```python
from build123d import *

# Parameters (mm, degrees)
F1_DEPTH = 20
F2_SIZE  = 5
F4_DEPTH = 25


with BuildPart() as f1:
    # F0 (on Top) → F1 (new body)
    with BuildSketch(Plane.XY):
        with BuildLine():
            Line((-45, 0), (0, 0))
            Line((0, 0), (0, 115))
            Line((0, 115), (-22, 115))
            ThreePointArc((-22, 115), (-24.12132, 115.87868), (-25, 118))
            Line((-25, 118), (-25, 120.717968))
            ThreePointArc((-25, 120.717968), (-38.514543, 135.644234), (-54.705789, 123.674277))
            ThreePointArc((-54.705789, 123.674277), (-55.961881, 121.238038), (-58.313624, 119.830085))
            Line((-58.313624, 119.830085), (-95, 110))
            Line((-95, 110), (-105, 110))
            Line((-105, 110), (-105, 100))
            ThreePointArc((-105, 100), (-97.928932, 97.071068), (-95, 90))
            ThreePointArc((-95, 90), (-97.928932, 82.928932), (-105, 80))
            Line((-105, 80), (-105, 70))
            Line((-105, 70), (-95, 70))
            ThreePointArc((-95, 70), (-91.464466, 68.535534), (-90, 65))
            Line((-90, 65), (-90, 45))
            Line((-90, 45), (-82.5, 45))
            ThreePointArc((-82.5, 45), (-75, 52.5), (-67.5, 45))
            ThreePointArc((-67.5, 45), (-69.696699, 39.696699), (-75, 37.5))
            Line((-75, 37.5), (-75, 30))
            ThreePointArc((-75, 30), (-64.393398, 25.606602), (-60, 15))
            Line((-60, 15), (-52.5, 15))
            ThreePointArc((-52.5, 15), (-45, 22.5), (-37.5, 15))
            ThreePointArc((-37.5, 15), (-39.696699, 9.696699), (-45, 7.5))
            Line((-45, 7.5), (-45, 0))
        make_face()
        with BuildLine():
            ThreePointArc((-47.5, 120.717968), (-40, 128.217968), (-32.5, 120.717968))
            ThreePointArc((-32.5, 120.717968), (-40, 113.217968), (-47.5, 120.717968))
        make_face(mode=Mode.SUBTRACT)
        with BuildLine():
            ThreePointArc((-105, 110), (-125, 90), (-105, 70))
            Line((-105, 70), (-105, 80))
            ThreePointArc((-105, 80), (-115, 90), (-105, 100))
            Line((-105, 100), (-105, 110))
        make_face()
        with BuildLine():
            ThreePointArc((-60, 15), (-55.606602, 4.393398), (-45, 0))
            Line((-45, 0), (-45, 7.5))
            ThreePointArc((-45, 7.5), (-50.303301, 9.696699), (-52.5, 15))
            Line((-52.5, 15), (-60, 15))
        make_face()
        with BuildLine():
            ThreePointArc((-90, 45), (-85.606602, 34.393398), (-75, 30))
            Line((-75, 30), (-75, 37.5))
            ThreePointArc((-75, 37.5), (-80.303301, 39.696699), (-82.5, 45))
            Line((-82.5, 45), (-90, 45))
        make_face()
    extrude(amount=F1_DEPTH)

    # F2
    f2_edges = [f1.edges().sort_by_distance(p)[0] for p in [
        (0, 115, 10),
        (0, 0, 10),
    ]]
    chamfer(f2_edges, length=F2_SIZE)

    # F3 (on face) → F4 (cut)
    with BuildSketch(Plane.XY.offset(20)):
        with BuildLine():
            Line((-45, 45), (-45, 37.5))
            ThreePointArc((-45, 37.5), (-42.129874, 38.070904), (-39.696699, 39.696699))
            Line((-39.696699, 39.696699), (-18.483496, 60.909903))
            ThreePointArc((-18.483496, 60.909903), (-18.483496, 71.516504), (-29.090097, 71.516504))
            Line((-29.090097, 71.516504), (-50.303301, 50.303301))
            ThreePointArc((-50.303301, 50.303301), (-51.929096, 47.870126), (-52.5, 45))
            Line((-52.5, 45), (-45, 45))
        make_face()
        with BuildLine():
            ThreePointArc((-52.5, 45), (-50.303301, 39.696699), (-45, 37.5))
            Line((-45, 37.5), (-45, 45))
            Line((-45, 45), (-52.5, 45))
        make_face()
    extrude(amount=-F4_DEPTH, mode=Mode.SUBTRACT)


solid = f1.part
```
Build history of the part. All positions in model axes, mm. A direction names the side the tool comes from. Coordinates: 2 decimals unless noted, no trailing zeros. Order: outer loops, then holes, each group sorted by start corner. A loop starts at its lowest first (then second) coordinate and runs counter-clockwise, first axis right, second up. Notation, with made-up numbers: (4.5, 22.25) -> (17.5, 22.25) arc R8 cw to (17.5, 29.25) -> close; hole circle Ø2 at (39.5, 37). An arc over 180 degrees is marked (long way). Answer in a Markdown table with one row per item. Add a question column.
Q1. Band-saw the part on C-C, the plane y = 108.5. List the corners of the cut face in (x, z).
Q2. Which spindle directions (+Z, -Z, +X, -X, +Y, -Y) get a long thin tool onto all of the face, cutting with end or side? Do faces 5 (the face through (-29.239, 50.155, 10.14)), 6 (the face through (-13, 115, 10)), 7 (the face through (-100, 110, 10)), 8 (the face through (-100, 70, 10)). Say none if no direction does.
Q3. Drop flat-ended pins along their axis: pin 1 (5 mm diameter, centred on x = -16, z = 13, fed in from +Y); pin 2 (5 mm diameter, centred on y = 55.5, z = 7.5, fed in from -X); pin 3 (12 mm diameter, centred on x = -40, y = 120.72, fed in from -Z); pin 4 (8 mm diameter, centred on x = -101.5, z = 10, fed in from +Y). Give the stop position or say it passes through.
Q4. Wall check: line 1 along X through (y, z) = (15.5, 4.25); line 2 along Y through (x, z) = (-40, 5.25); line 3 along X through (y, z) = (40, 8.25). Give the ranges that are in metal, low to high. Write a range as [from, to].
Q5. Band-saw the part on B-B, the plane y = 85.5. List the corners of the cut face in (x, z).
Q6. Mould opens along Y. For faces 1 (the face through (-49, 69, 20)), 2 (the face through (-25, 0, 10)), 3 (the face through (-76.4, 114.984, 9.86)), 4 (the face through (-39.548, 61.058, 10.14)) say: +Y half, -Y half, draft (parallel to the pull), parting line (faces both ways), or undercut.
Q7. Band-saw the part on A-A, the plane z = 5.25. Give the number of separate pieces and of enclosed holes in the cut face, then the cut area to 3 significant figures.
Answers follow:
| question | item | result |
|---|---|---|
| 1 | outline | (-112.6, 0) -> (0, 0) -> (0, 20) -> (-112.6, 20) -> close |
| 2 | face 5 | +Z, -Z |
| 2 | face 6 | +Z, -Z, +X, +Y |
| 2 | face 7 | +Z, -Z, -X, +Y |
| 2 | face 8 | +Z, -Z, -X, -Y |
| 3 | pin 1 | y = 115 |
| 3 | pin 2 | x = -90 |
| 3 | pin 3 | through |
| 3 | pin 4 | y = 110 |
| 4 | line 1 | [-60.01, -52.48], [-37.52, 0] |
| 4 | line 2 | [0, 9.41], [20.59, 39.41], [60.61, 113.22], [128.22, 135.72] |
| 4 | line 3 | [-89.14, -80.59], [-69.41, -50.59], [-39.39, 0] |
| 5 | outline | (-124.49, 0) -> (-113.93, 0) -> (-113.93, 20) -> (-124.49, 20) -> close; (-96.07, 0) -> (0, 0) -> (0, 20) -> (-96.07, 20) -> close |
| 6 | face 1 | draft |
| 6 | face 2 | -Y half |
| 6 | face 3 | +Y half |
| 6 | face 4 | undercut |
| 7 | separate pieces | 1 |
| 7 | enclosed holes | 5 |
| 7 | area | 9,710 mm^2 |
